Geometry: final body of the model. Coordinates: model frame, mm. A direction names the side the tool comes from. Give positions to 0.01 mm unless a question says otherwise; leave off trailing zeros. Write each loop counter-clockwise with the first axis right and the second up, starting at its lowest first coordinate (ties: lowest second). Pieces come first, ordered by that corner, then holes. Notation, with made-up numbers: (32, -22.75) -> (48, -22.75) arc R16 ccw to (48, 4.25) -> close; hole circle Ø3 at (83, -18.5). An arc over 180 degrees is marked (long way). Use CSV: the item, a comma, the result in double quotes. Start each with the question number.
1) Contact query for flat-ended pins moving along their axis: P1, Ø1.5, axis at y = 23.5, z = 11, coming from the -X side; P2, Ø7.5, axis at x = 1.5, z = 313.5, coming from the +Y side; P3, Ø3, axis at x = 1.5, y = 19.5, coming from the +Z side. Output: stop coordinate, or through.
2) Section A-A (z = 83). Output: boundary loops of the cut face in (x, y).
3) Material intervals for line 1 (X direction, y = -5.5, z = 295); line 2 (Y direction, x = 9, z = 221.5), sorted ascending. Write a range as [from, to].
4) Set-up query: faces 1 (the face through (0, -12.5, 246)), 2 (the face through (-7.5, 0, 246)). Return all of +Z, -Z, +X, -X, +Y, -Y with unobstructed straight access to the full face (end or side cutting, diameter ignored); none if empty.
5) Draft query along Z for faces 3 (the face through (-1.72, -10.04, 66.83)), 4 (the face through (-9, 0, 0)), 5 (the face through (0, 22, 12.731)), 6 (the face through (0, 32.5, 8)). Return one class per face: pulls with the +Z half, pulls with the -Z half, needs draft (parallel to the pull), parting line crosses it, or undercut.
```python
from build123d import *

# Parameters (mm, degrees)
SKETCH1_W           = 25
SKETCH1_H           = 25
SKETCH1_W_2         = 15
SKETCH1_H_2         = 15
BOSS_EXTRUDE1_DEPTH = 500
SKETCH2_W           = 10
SKETCH2_H           = 10
BOSS_EXTRUDE2_DEPTH = 20
SKETCH3_R           = 2.5
BOSS_EXTRUDE3_DEPTH = 20
FILLET2_R           = 5
FILLET3_R           = 5
SKETCH4_R           = 4.5
CUT_EXTRUDE1_DEPTH  = 5


with BuildPart() as part:
    # Sketch1 → Boss-Extrude1 (new body)
    with BuildSketch(Plane.XY):
        Rectangle(SKETCH1_W, SKETCH1_H)
        Rectangle(SKETCH1_W_2, SKETCH1_H_2, mode=Mode.SUBTRACT)
    extrude(amount=BOSS_EXTRUDE1_DEPTH)

    # Sketch2 → Boss-Extrude2 (add)
    with BuildSketch(Plane(origin=(0, 12.5, 0), x_dir=(1, 0, 0), z_dir=(0, 1, 0))):
        with Locations((0, -7.731161073)):
            Rectangle(SKETCH2_W, SKETCH2_H)
    extrude(amount=BOSS_EXTRUDE2_DEPTH)

    # Sketch3 → Boss-Extrude3 (add)
    with BuildSketch(Plane.XY.offset(12.731161073)):
        with Locations(Location((0, 27.707080849, 0), (0, 0, 180))):
            Circle(SKETCH3_R)
    extrude(amount=BOSS_EXTRUDE3_DEPTH)

    # Fillet2
    fillet2_edges = [part.edges().sort_by_distance(p)[0] for p in [
        (5, 22.5, 2.731161073),
    ]]
    fillet(fillet2_edges, radius=FILLET2_R)

    # Fillet3
    fillet3_edges = [part.edges().sort_by_distance(p)[0] for p in [
        (-5, 22.5, 2.731161073),
    ]]
    fillet(fillet3_edges, radius=FILLET3_R - 0.0001)  # a hair under: the kernel refuses the full size

    # Sketch4 → Cut-Extrude1 (cut)
    with BuildSketch(Plane.XZ.offset(12.5)):
        with Locations(Location((0, 70.986744053, 0), (0, 0, 270))):
            Circle(SKETCH4_R)
    extrude(amount=-CUT_EXTRUDE1_DEPTH, mode=Mode.SUBTRACT)


solid = part.part
```
Answers follow:
1,P1,"stops at x = -5"
1,P2,"stops at y = 12.5"
1,P3,"stops at z = 12.73"
2,outline,"(-12.5, -12.5) -> (12.5, -12.5) -> (12.5, 12.5) -> (-12.5, 12.5) -> close; hole (-7.5, -7.5) -> (7.5, -7.5) -> (7.5, 7.5) -> (-7.5, 7.5) -> close"
3,line 1,"x = [-12.5, -7.5], [7.5, 12.5]"
3,line 2,"y = [-12.5, 12.5]"
4,face 1,"+Z, -Z, +X, -X, -Y"
4,face 2,"+Z, -Z"
5,face 3,"undercut"
5,face 4,"pulls with the -Z half"
5,face 5,"pulls with the +Z half"
5,face 6,"needs draft"
